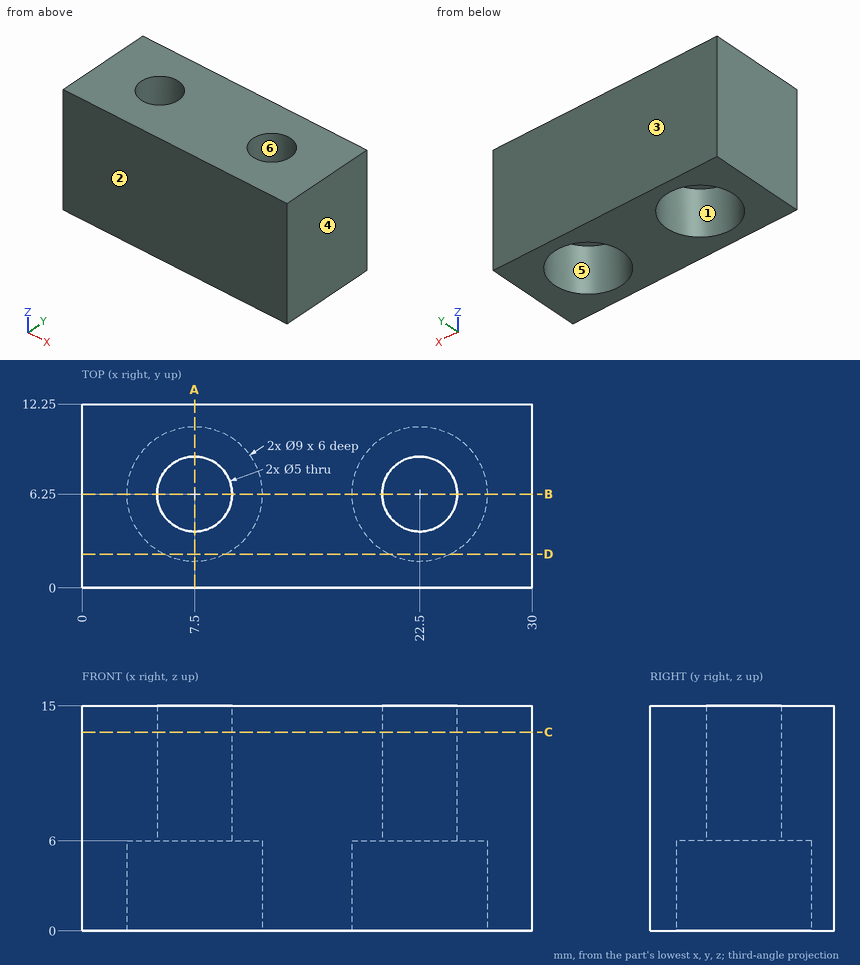
Could you check a few things on this drawing? It's one solid part, dimensions in mm from its lowest x, y, z. A direction names the side the tool comes from. Give positions to 0.01 mm unless a question says otherwise; leave off trailing zeros. Write each loop counter-clockwise with the first axis right and the second up, starting at its lowest first coordinate (ties: lowest second). Pieces come first, ordered by that corner, then holes. Notation, with made-up numbers: (-21.75, 52.5) -> (-3.75, 52.5) arc R9 cw to (-3.75, 57.5) -> close; hole circle Ø10 at (-23.75, 49.25). An arc over 180 degrees is marked (long way). Answer as a JSON object with one key per item and string values.
Q1. Suppose I cut it at D-D on y = 2.25. Write out the boundary of the cut face in (x, z), then the cut area to 3 significant figures.
Taken from the geometry:
{"outline": "(0, 0) -> (5.44, 0) -> (5.44, 6) -> (9.56, 6) -> (9.56, 0) -> (20.44, 0) -> (20.44, 6) -> (24.56, 6) -> (24.56, 0) -> (30, 0) -> (30, 15) -> (0, 15) -> close", "area": "401 mm²"}
Q2. Suppose I cut it at B-B on y = 6.25. Write out the boundary of the cut face in (x, z).
Taken from the geometry:
{"outline": "(0, 0) -> (3, 0) -> (3, 6) -> (5, 6) -> (5, 15) -> (0, 15) -> close; (10, 6) -> (12, 6) -> (12, 0) -> (18, 0) -> (18, 6) -> (20, 6) -> (20, 15) -> (10, 15) -> close; (25, 6) -> (27, 6) -> (27, 0) -> (30, 0) -> (30, 15) -> (25, 15) -> close"}
Q3. Which directions (+Z, -Z, +X, -X, +Y, -Y) give clear straight access to the entire face, cutting with the end or side of a thin tool? Please do the marked faces 5 and 6.
Taken from the geometry:
{"face 5": "-Z", "face 6": "+Z, -Z"}
Q4. We'd pull the mould along Y, two halves only. Please class the marked faces 1, 2, 3 and 4: released by +Y, released by -Y, zero draft, split by the parting line, or undercut.
Taken from the geometry:
{"face 1": "undercut", "face 2": "released by -Y", "face 3": "released by +Y", "face 4": "zero draft"}
Q5. Will these pins go through, and if not, where does the flat tip stop? pin 1 Ø6.5 at (x, y) = (7.5, 6.25) entering from -Z; pin 2 Ø1 at (y, z) = (1.5, 3.5) entering from -X.
Taken from the geometry:
{"pin 1": "stops at z = 6", "pin 2": "stops at x = 0"}
Q6. Suppose I cut it at A-A on x = 7.5. Write out the boundary of the cut face in (y, z), then the cut area to 4 significant figures.
Taken from the geometry:
{"outline": "(0, 0) -> (1.75, 0) -> (1.75, 6) -> (3.75, 6) -> (3.75, 15) -> (0, 15) -> close; (8.75, 6) -> (10.75, 6) -> (10.75, 0) -> (12.25, 0) -> (12.25, 15) -> (8.75, 15) -> close", "area": "84.75 mm²"}
Q7. Suppose I cut it at C-C on z = 13.25. Write out the boundary of the cut face in (x, y), then the cut area to 3 significant figures.
Taken from the geometry:
{"outline": "(0, 0) -> (30, 0) -> (30, 12.25) -> (0, 12.25) -> close; hole circle Ø5 at (7.5, 6.25); hole circle Ø5 at (22.5, 6.25)", "area": "328 mm²"}
Q8. Please list where these lines run through material, in increasing order: L1, parallel to X at y = 6.25, z = 8.5; L2, parallel to Y at x = 22.5, z = 3.55; L3, parallel to X at y = 2.75, z = 3.
Taken from the geometry:
{"L1": "x = 0 to 5, 10 to 20, 25 to 30", "L2": "y = 0 to 1.75, 10.75 to 12.25", "L3": "x = 0 to 4.67, 10.33 to 19.67, 25.33 to 30"}
